```python
from build123d import *

# Parameters (mm, degrees)
SKETCH1_W     = 1.5875
SKETCH1_H     = 161.737331671
CHAMFER1_SIZE = 0.254


with BuildPart() as part:
    # Sketch1 → Revolve1 (revolve)
    with BuildSketch(Plane.XY):
        with Locations((5.55625, 205.12785438)):
            Rectangle(SKETCH1_W, SKETCH1_H)
    revolve(axis=Axis((0, 114.734188544, 0), (0, 1, 0)))

    # Chamfer1
    chamfer1_edges = [part.edges().sort_by_distance(p)[0] for p in [
        (-6.35, 124.259188544, 0),
        (-6.349999999, 285.996520215, 0),
        (-4.762499999, 285.996520215, 0),
        (-4.7625, 124.259188544, 0),
    ]]
    chamfer(chamfer1_edges, length=CHAMFER1_SIZE)


solid = part.part
```
Input: part model. Units: mm. Frame: model coordinates. Give positions to 0.01 mm unless a question says otherwise; leave off trailing zeros. Order: outer loops, then holes, each group sorted by start corner. A loop starts at its lowest first (then second) coordinate and runs counter-clockwise, first axis right, second up. Notation, with made-up numbers: (80, -31.5) -> (137, -31.5) arc R21 ccw to (137, -1.5) -> close; hole circle Ø11 at (75.5, 14). An arc over 180 degrees is marked (long way). Write each question's results on one line, items separated by ' | '. Start each with the question number.
Item 1: Line query: line 1 (X direction, y = 237.5, z = 0); line 2 (Z direction, x = -0.5, y = 274). Output: solid intervals per line, ascending.
Item 2: Cut plane A-A on x = 0. Return the cut outline in (y, z).
Item 3: Cut plane B-B on z = 0. Return the cut outline in (x, y).
Item 4: Mould query, pull axis X, two halves, no side actions, for faces 1 (the flat face through (5, 285.997, -2)), 2 (the cylindrical face through (-3.78, 206.26, 2.9)), 3 (the cylindrical face through (-0.8, 206.3, -6.3)). Classes: pulls with the +X half, pulls with the -X half, needs draft (parallel to the pull), parting line crosses it, or undercut.
Item 5: Contact query for flat-ended pins moving along their axis: P1, Ø4, axis at x = -1, z = -2.5, coming from the -Y side; P2, Ø5, axis at x = -3, z = -2, coming from the +Y side. Output: stop coordinate, or through.
Established:
1) line 1: -6.35 to -4.76, 4.76 to 6.35 | line 2: -6.33 to -4.74, 4.74 to 6.33
2) outline: (124.26, -6.1) -> (124.51, -6.35) -> (285.74, -6.35) -> (286, -6.1) -> (286, -5.02) -> (285.74, -4.76) -> (124.51, -4.76) -> (124.26, -5.02) -> close; (124.26, 5.02) -> (124.51, 4.76) -> (285.74, 4.76) -> (286, 5.02) -> (286, 6.1) -> (285.74, 6.35) -> (124.51, 6.35) -> (124.26, 6.1) -> close
3) outline: (-6.35, 124.51) -> (-6.1, 124.26) -> (-5.02, 124.26) -> (-4.76, 124.51) -> (-4.76, 285.74) -> (-5.02, 286) -> (-6.1, 286) -> (-6.35, 285.74) -> close; (4.76, 124.51) -> (5.02, 124.26) -> (6.1, 124.26) -> (6.35, 124.51) -> (6.35, 285.74) -> (6.1, 286) -> (5.02, 286) -> (4.76, 285.74) -> close
4) face 1: needs draft | face 2: undercut | face 3: parting line crosses it
5) P1: through | P2: y = 286
